Design review of the part built by this model. Coordinates are the model's own, in mm. Face numbers are marked on the shaded views. A direction names the side the tool comes from. Coordinates: 2 decimals unless noted, no trailing zeros. Write each loop counter-clockwise with the first axis right and the second up, starting at its lowest first coordinate (ties: lowest second). Pieces come first, ordered by that corner, then holes. Notation, with made-up numbers: (82.5, 7.5) - (125.5, 7.5) arc R18 cw to (125.5, 35.5) - close; hole circle Ø5 at (19.25, 53). An arc over 180 degrees is marked (long way). Use a Markdown table: item, result.
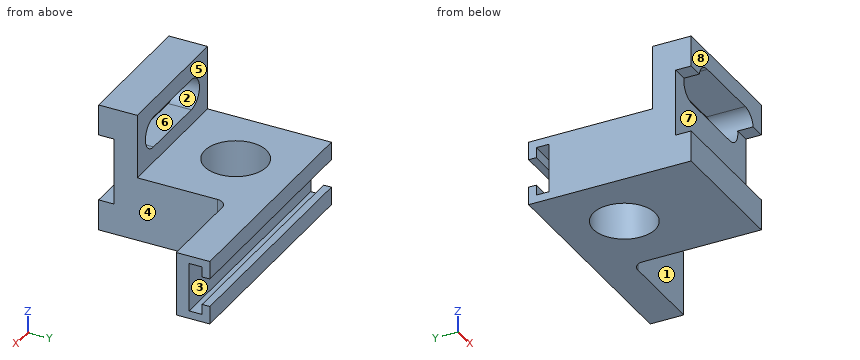
from build123d import *

# Parameters (mm, degrees)
BOSS_EXTRUDE3_DEPTH = 50
SKETCH1_5_W         = 104
SKETCH1_5_H         = 30
BOSS_EXTRUDE4_DEPTH = 100
SKETCH4_W           = 52
SKETCH4_H           = 12
CUT_EXTRUDE1_DEPTH  = 242.404225315
CUT_EXTRUDE2_DEPTH  = 242.404225315
CUT_EXTRUDE3_DEPTH  = 228.191549139
SKETCH7_R           = 24
CUT_EXTRUDE4_DEPTH  = 226.335305711
FILLET3_R           = 8


with BuildPart() as part:
    # Sketch1 → Boss-Extrude3 (new body)
    with BuildSketch(Plane.XY):
        Polygon((0, 126), (0, 30), (104, 30), (104, 100), (180, 100), (180, 126), align=None)
    extrude(amount=BOSS_EXTRUDE3_DEPTH)

    # Sketch1<5> → Boss-Extrude4 (add)
    with BuildSketch(Plane.XY):
        with Locations((52, 15)):
            Rectangle(SKETCH1_5_W, SKETCH1_5_H)
    extrude(amount=BOSS_EXTRUDE4_DEPTH)

    # Sketch4 → Cut-Extrude1 (cut, through all)
    with BuildSketch(Plane(origin=(180, 0, 0), x_dir=(0, 0, -1), z_dir=(1, 0, 0))):
        with Locations((-50, 6)):
            Rectangle(SKETCH4_W, SKETCH4_H)
    extrude(amount=-CUT_EXTRUDE1_DEPTH, mode=Mode.SUBTRACT)

    # Sketch4<5> → Cut-Extrude2 (cut, through all)
    with BuildSketch(Plane(origin=(180, 0, 0), x_dir=(0, 0, -1), z_dir=(1, 0, 0))):
        Polygon((-36, 126), (-36, 120), (-44, 120), (-44, 110), (-6, 110), (-6, 120), (-14, 120), (-14, 126), align=None)
    extrude(amount=-CUT_EXTRUDE2_DEPTH, mode=Mode.SUBTRACT)

    # Sketch5 → Cut-Extrude3 (cut, through all)
    with BuildSketch(Plane(origin=(0, 30, 0), x_dir=(1, 0, 0), z_dir=(0, 1, 0))):
        with BuildLine():
            Line((24, -62), (80, -62))
            ThreePointArc((80, -62), (92, -74), (80, -86))
            Line((80, -86), (24, -86))
            ThreePointArc((24, -86), (12, -74), (24, -62))
        make_face()
    extrude(amount=-CUT_EXTRUDE3_DEPTH, mode=Mode.SUBTRACT)

    # Sketch7 → Cut-Extrude4 (cut, through all)
    with BuildSketch(Plane.XY.offset(50)):
        with Locations((50, 78)):
            Circle(SKETCH7_R)
    extrude(amount=-CUT_EXTRUDE4_DEPTH, mode=Mode.SUBTRACT)

    # Fillet3
    fillet3_edges = [part.edges().sort_by_distance(p)[0] for p in [
        (104, 100, 25),
    ]]
    fillet(fillet3_edges, radius=FILLET3_R)


solid = part.part
(1) Draft analysis for pull direction Y (two halves, no side actions). For the marked faces 1, 2 and 3, state which applies: +Y half, -Y half, draft (parallel to the pull), parting line (faces both ways), or undercut.
Determined:
| item | result |
|---|---|
| face 1 | -Y half |
| face 2 | draft |
| face 3 | undercut |
(2) Take a section at A-A on y = 78. Write out the cut boundary in (x, z), and give its area (3 significant figures).
Determined:
| item | result |
|---|---|
| outline | (0, 0) - (26, 0) - (26, 50) - (0, 50) - close; (74, 0) - (104, 0) - (104, 50) - (74, 50) - close |
| area | 2,800 mm2 |
(3) For pin 1 (6.5 mm diameter, centred on x = 60, y = 124, fed in from +Z); pin 2 (3 mm diameter, centred on x = 84.5, y = 124.5, fed in from -Z); pin 3 (15 mm diameter, centred on x = 37.5, z = 76, fed in from +Y); pin 4 (2.5 mm diameter, centred on x = 88, z = 41.5, fed in from -Y), all flat-tipped, find the tip position at first contact; note any pin that passes through.
Determined:
| item | result |
|---|---|
| pin 1 | z = 50 |
| pin 2 | z = 0 |
| pin 3 | through |
| pin 4 | y = 12 |
(4) Take a section at C-C on x = 50. Write out the cut boundary in (y, z).
Determined:
| item | result |
|---|---|
| outline | (0, 0) - (54, 0) - (54, 50) - (30, 50) - (30, 62) - (12, 62) - (12, 24) - (0, 24) - close; (0, 86) - (30, 86) - (30, 100) - (0, 100) - close; (102, 0) - (126, 0) - (126, 14) - (120, 14) - (120, 6) - (110, 6) - (110, 44) - (120, 44) - (120, 36) - (126, 36) - (126, 50) - (102, 50) - close |
(5) Machinability: for the marked faces 4, 5, 6, 7 and 8, which of the approach directions +Z, -Z, +X, -X, +Y, -Y give a long, thin tool a straight path to every point of the face, cutting with its end or side? Answer none if there is none.
Determined:
| item | result |
|---|---|
| face 4 | +Z, -Z, +X, -Y |
| face 5 | +Z, +X, -X, +Y |
| face 6 | +Y, -Y |
| face 7 | +X, -X, -Y |
| face 8 | +Z, -Z, +X, -X, -Y |
(6) For L1, parallel to Y at x = 50, z = 10.5; L2, parallel to Y at x = 50, z = 21; L3, parallel to Y at x = 130, z = 43.5, list the stretches that pass through material, from the lowest coordinate up. Write a range as from..to.
Determined:
| item | result |
|---|---|
| L1 | 0..54, 102..110, 120..126 |
| L2 | 0..54, 102..110 |
| L3 | 100..110, 120..126 |
(7) Take a section at B-B on z = 74. Write out the cut boundary in (x, y).
Determined:
| item | result |
|---|---|
| outline | (0, 12) - (12, 12) - (12, 30) - (0, 30) - close; (92, 12) - (104, 12) - (104, 30) - (92, 30) - close |
(8) Take a section at D-D on y = 28. Write out the cut boundary in (x, z), and give its area (3 significant figures).
Determined:
| item | result |
|---|---|
| outline | (0, 0) - (104, 0) - (104, 100) - (0, 100) - close; hole (24, 62) - (80, 62) arc R12 ccw to (80, 86) - (24, 86) arc R12 ccw to start |
| area | 8,600 mm2 |
